```python
from build123d import *

# Parameters (mm, degrees)
SALIENTE_EXTRUIR1_DEPTH = 7
CROQUIS2_R              = 2.4
CORTAR_EXTRUIR1_DEPTH   = 5
CORTAR_EXTRUIR2_DEPTH   = 8
CROQUIS4_W              = 4
CROQUIS4_H              = 37.728244425
CORTAR_EXTRUIR3_DEPTH   = 40
SALIENTE_EXTRUIR2_DEPTH = 8


with BuildPart() as part:
    # Croquis1 → Saliente-Extruir1 (new body)
    with BuildSketch(Plane.XY):
        with BuildLine():
            Line((-58.064516129, 28.516129032), (-50.064516129, 28.516129032))
            Line((-50.064516129, 28.516129032), (-50.064516129, 17.972961327))
            ThreePointArc((-50.064516129, 17.972961327), (-39.064516129, 3.516129032), (-50.064516129, -10.940703263))
            Line((-50.064516129, -10.940703263), (-50.064516129, -21.483870968))
            Line((-50.064516129, -21.483870968), (-58.064516129, -21.483870968))
            Line((-58.064516129, -21.483870968), (-58.064516129, -10.940703263))
            ThreePointArc((-58.064516129, -10.940703263), (-69.064516129, 3.516129032), (-58.064516129, 17.972961327))
            Line((-58.064516129, 17.972961327), (-58.064516129, 28.516129032))
        make_face()
    extrude(amount=SALIENTE_EXTRUIR1_DEPTH)

    # Croquis2 → Cortar-Extruir1 (cut)
    with BuildSketch(Plane.XZ.offset(21.483870968)):
        with Locations(Location((-54.064516129, 3.5, 0), (0, 0, 270))):
            Circle(CROQUIS2_R)
    extrude(amount=-CORTAR_EXTRUIR1_DEPTH, mode=Mode.SUBTRACT)

    # Croquis3 → Cortar-Extruir2 (cut)
    with BuildSketch(Plane.ZY.offset(58.064516129)):
        Polygon((7, 24.516129032), (0, 28.516129032), (7, 28.516129032), align=None)
    extrude(amount=-CORTAR_EXTRUIR2_DEPTH, mode=Mode.SUBTRACT)

    # Croquis4 → Cortar-Extruir3 (cut)
    with BuildSketch(Plane.ZY.offset(69.064516129)):
        with Locations((2, 5.007952278)):
            Rectangle(CROQUIS4_W, CROQUIS4_H)
    extrude(amount=-CORTAR_EXTRUIR3_DEPTH, mode=Mode.SUBTRACT)

    # Croquis5 → Saliente-Extruir2 (add)
    with BuildSketch(Plane.ZY.offset(58.064516129)):
        Polygon((0, 23.87207449), (4, 17.972961327), (4, 23.87207449), align=None)
        Polygon((0, -13.856169935), (4, -10.940703263), (4, -13.856169935), align=None)
    extrude(amount=-SALIENTE_EXTRUIR2_DEPTH)


solid = part.part
```
The listing builds one solid part. Answer for the finished solid, in the listing's coordinates (mm). A direction names the side the tool comes from. Coordinates: 2 decimals unless noted, no trailing zeros. Loops run counter-clockwise (first coordinate to the right, second up) from the corner with the lowest first, then second, coordinate; pieces in that order, holes last. Notation, with made-up numbers: (-27.5, 80.25) -> (9.5, 80.25) arc R12 cw to (9.5, 90.25) -> close; hole circle Ø3 at (39, 61). An arc over 180 degrees is marked (long way). Return JSON: item names as keys, results as strings. Group by question number.
(1) Given pin 1 Ø4 at (x, y) = (-65.5, 6) entering from -Z; pin 2 Ø1.4 at (x, z) = (-54, 2.5) entering from -Y; pin 3 Ø3.5 at (y, z) = (-17.5, 4.5) entering from +X, each flat-ended and moving along its own axis, determine where each tip first touches the part or whether it passes through.
(2) Determine the mould class of faces 5 (the flat face through (-54, -16.484, 4)), 6 (the flat face through (-50.065, 23, 3)), 7 (the cylindrical face through (-56.194, -19.019, 2.393)), 8 (the flat face through (-54, 26, 0)) for opening direction X: released by +X, released by -X, zero draft, split by the parting line, or undercut.
(3) A cutting plane is placed at B-B on x = -45.25. Write down the section's boundary in (y, z), and give its area (3 significant figures).
(4) A cutting plane is placed at A-A on z = 2.5. Write down the section's boundary in (x, y), and give its area (3 significant figures).
(5) A cutting plane is placed at C-C on y = 11. Write down the section's boundary in (x, z).
(6) Which of the six approach directions +Z, -Z, +X, -X, +Y, -Y give full straight-line access (tool end or side, diameter ignored) to faces 1 (the flat face through (-54.121, 20.964, 1.972)), 2 (the flat face through (-58.065, -16, 3)), 3 (the flat face through (-50.065, -16, 3)), 4 (the flat face through (-58.065, 23, 3))?
(7) Find the intervals of material crossed by probe 1 along X at (y, z) = (-18.5, 3.5); probe 2 along Z at (x, y) = (-56.5, 8.5); probe 3 along Y at (x, z) = (-54.25, 0.75), in increasing order. Write a range as from..to.
The answers:
{
 "1": {"pin 1": "stops at z = 4", "pin 2": "stops at y = -16.48", "pin 3": "stops at x = -50.06"},
 "2": {"face 5": "undercut", "face 6": "released by +X", "face 7": "undercut", "face 8": "zero draft"},
 "3": {"outline": "(-8.62, 4) -> (15.65, 4) -> (15.65, 7) -> (-8.62, 7) -> close", "area": "72.8 mm^2"},
 "4": {"outline": "(-58.06, -21.48) -> (-56.25, -21.48) -> (-56.25, -16.48) -> (-51.88, -16.48) -> (-51.88, -21.48) -> (-50.06, -21.48) -> (-50.06, -12.03) -> (-58.06, -12.03) -> close; (-58.06, 20.19) -> (-50.06, 20.19) -> (-50.06, 27.09) -> (-58.06, 27.09) -> close", "area": "109 mm^2"},
 "5": {"outline": "(-67.06, 4) -> (-41.06, 4) -> (-41.06, 7) -> (-67.06, 7) -> close"},
 "6": {"face 1": "-Z, +X, -X", "face 2": "+Z, -Z, -X, -Y", "face 3": "+Z, -Z, +X, -Y", "face 4": "+Z, -Z, -X, +Y"},
 "7": {"probe 1": "x = -58.06..-56.46, -51.66..-50.06", "probe 2": "z = 4..7", "probe 3": "y = -21.48..-13.31, 22.77..28.09"}
}
